Geometry: see drawing. Coordinates: mm, zero at the bounding-box minimum. Round coordinates to 2 decimals unless told otherwise and drop trailing zeros. Write each loop counter-clockwise with the first axis right and the second up, starting at its lowest first coordinate (ties: lowest second). Pieces come first, ordered by that corner, then holes.
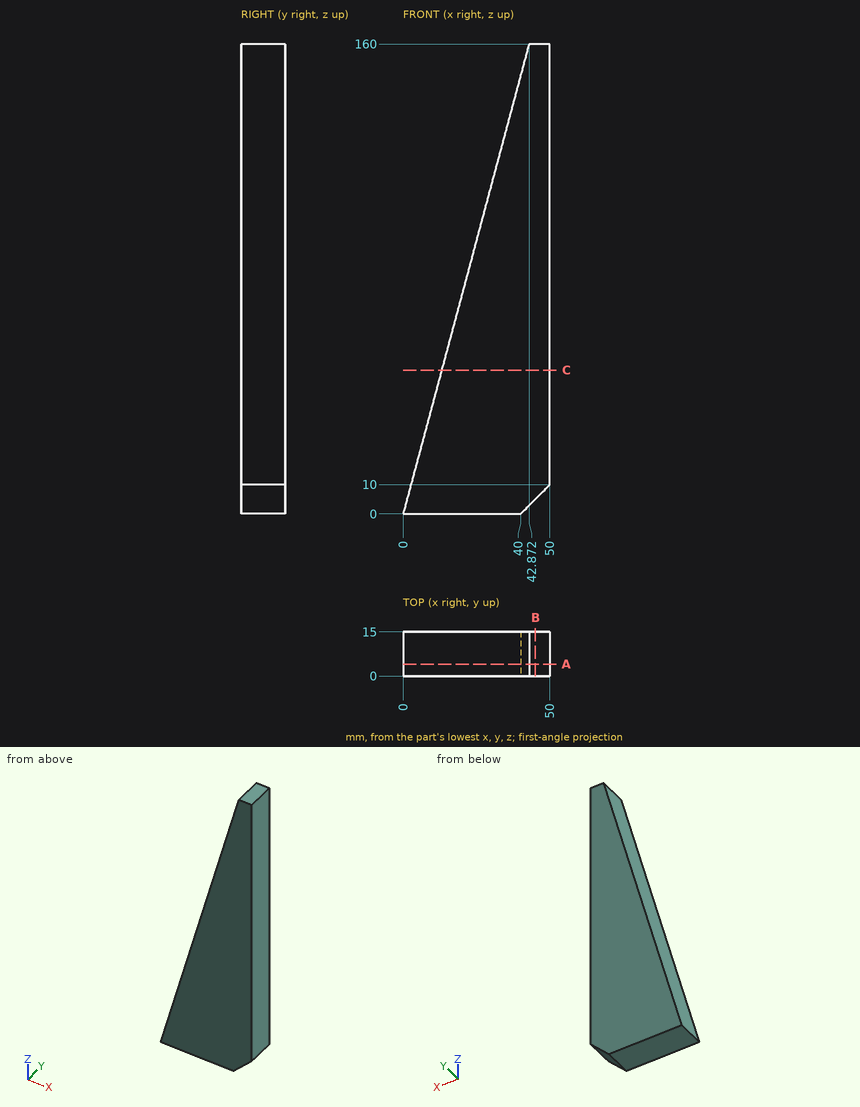
1) Section query B-B on x = 45. Return the cut outline in (y, z), then the cut area to 4 significant figures.
Taken from the geometry:
outline: (0, 5) - (15, 5) - (15, 160) - (0, 160) - close
area: 2,325 mm2
2) Material intervals for line 1 (X direction, y = 10.5, z = 70); line 2 (X direction, y = 3.5, z = 32), sorted ascending.
Taken from the geometry:
line 1: x = 18.76 to 50
line 2: x = 8.57 to 50
3) Section query A-A on y = 4. Return the cut outline in (x, z).
Taken from the geometry:
outline: (0, 0) - (40, 0) - (50, 10) - (50, 160) - (42.87, 160) - close
4) Section query C-C on z = 49. Return the cut outline in (x, y), then the cut area to 3 significant figures.
Taken from the geometry:
outline: (13.13, 0) - (50, 0) - (50, 15) - (13.13, 15) - close
area: 553 mm2
5) Contact query for flat-ended pins moving along their axis: P1, Ø1.5, axis at y = 5.5, z = 26.5, coming from the -X side; P2, Ø3, axis at y = 8, z = 104, coming from the -X side (3 decimals). Output: stop coordinate, or through.
Taken from the geometry:
P1: stops at x = 6.9
P2: stops at x = 27.465
